Solid Edge part; units mm, degrees
sketch "Sketch1" plane through (0, 0, 0) normal (0, 0, 1) x (1, 0, 0)
  arc A0 (0, 5.3) -> (0.3, 5) centre (0.3, 5.3) ccw
  line L0 (0.3, 5) -> (6.7, 5)
  arc A1 (6.7, 5) -> (7, 5.3) centre (6.7, 5.3) ccw
  line L1 (7, 5.3) -> (7, 6.25)
  arc A2 (7, 6.25) -> (6.9, 6.35) centre (6.9, 6.25) ccw
  line L2 (6.9, 6.35) -> (4.2785, 6.35)
  arc A3 (4.2785, 6.35) -> (2.7215, 6.35) centre (3.5, 7.25) cw
  line L3 (2.7215, 6.35) -> (0.1, 6.35)
  arc A4 (0.1, 6.35) -> (0, 6.25) centre (0.1, 6.25) ccw
  line L4 (0, 6.25) -> (0, 5.3)
revolve "RevolvedProtrusion1" add sketch "Sketch1" angle 360 about axis through (6.7, 0, 0) along (-1, 0, 0)
sketch "Sketch2" plane through (0, 0, 0) normal (0, 0, 1) x (1, 0, 0)
  line L0 (0, 5.9) -> (0.324, 5.9)
  arc A0 (0.324, 5.9) -> (0.648, 6.224) centre (0.324, 6.224) ccw
  line L1 (0.648, 6.224) -> (0.648, 6.8)
  line L2 (0.648, 6.8) -> (6.352, 6.8)
  line L3 (6.352, 6.8) -> (6.352, 6.224)
  arc A1 (6.352, 6.224) -> (6.676, 5.9) centre (6.676, 6.224) ccw
  line L4 (6.676, 5.9) -> (7, 5.9)
  line L5 (7, 5.9) -> (7, 7.25)
  line L6 (7, 7.25) -> (0, 7.25)
  line L7 (0, 7.25) -> (0, 5.9)
revolve "RevolvedCutout1" cut sketch "Sketch2" angle 360 about axis through (7, 0, 0) along (-1, 0, 0)
Work out the finished part from the listing and answer in its coordinate system (mm). A direction names the side the tool comes from. Round coordinates to 2 decimals unless told otherwise and drop trailing zeros. Write each loop counter-clockwise with the first axis right and the second up, starting at its lowest first coordinate (ties: lowest second). Pieces come first, ordered by that corner, then holes.
1) Consider probe 1 along Y at (x, z) = (5.5, 0); probe 2 along Z at (x, y) = (4, 0). Determine where each line is inside the solid, lowest interval first.
2) Which of the six approach directions +Z, -Z, +X, -X, +Y, -Y give full straight-line access (tool end or side, diameter ignored) to faces 1 (the face through (5.3, -1.38, 6.2)), 2 (the face through (6.84, -5.894, 0.259)), 3 (the face through (0.164, -5.894, 0.259))?
3) A cutting plane is placed at C-C on x = 1.25. Determine the outline of the cut face in (y, z).
4) A cutting plane is placed at D-D on x = 4. Determine the outline of the cut face in (y, z).
5) A cutting plane is placed at A-A on z = 0. Determine the outline of the cut face in (x, y).
6) Determine the mould class of faces 4 (the face through (1.67, 5.866, 2.432)), 5 (the face through (3.54, -1.08, -4.88)), 6 (the face through (7, -4, -4)) for opening direction Y: pulls with the +Y half, pulls with the -Y half, needs draft (parallel to the pull), parting line crosses it, or undercut.
7) Flat-ended cylindrical pins translate along their axes: P1, Ø4, axis at y = 2.5, z = -2, coming from the -X side; P2, Ø1.5, axis at y = -4.5, z = -4, coming from the +X side; P3, Ø1.5, axis at x = 6, y = 1, coming from the +Z side. Find the tip coordinate at first contact, or state that the pin passes through.
Entries:
1. probe 1: y = -6.35 to -5, 5 to 6.35
1. probe 2: z = -6.17 to -5, 5 to 6.17
2. face 1: +X, -X
2. face 2: +X
2. face 3: -X
3. outline: circle Ø12.7 at (0, 0); hole circle Ø10 at (0, 0)
4. outline: circle Ø12.34 at (0, 0); hole circle Ø10 at (0, 0)
5. outline: (0, -5.9) - (0.32, -5.9) arc R0.32 cw to (0.65, -6.22) - (0.65, -6.35) - (2.72, -6.35) arc R1.19 cw to (4.28, -6.35) - (6.35, -6.35) - (6.35, -6.22) arc R0.32 cw to (6.68, -5.9) - (7, -5.9) - (7, -5.3) arc R0.3 ccw to (6.7, -5) - (0.3, -5) arc R0.3 ccw to (0, -5.3) - close; (0, 5.3) arc R0.3 ccw to (0.3, 5) - (6.7, 5) arc R0.3 ccw to (7, 5.3) - (7, 5.9) - (6.68, 5.9) arc R0.32 cw to (6.35, 6.22) - (6.35, 6.35) - (4.28, 6.35) arc R1.19 cw to (2.72, 6.35) - (0.65, 6.35) - (0.65, 6.22) arc R0.32 cw to (0.32, 5.9) - (0, 5.9) - close
6. face 4: parting line crosses it
6. face 5: undercut
6. face 6: needs draft
7. P1: stops at x = 0.02
7. P2: stops at x = 7
7. P3: stops at z = 6.35
